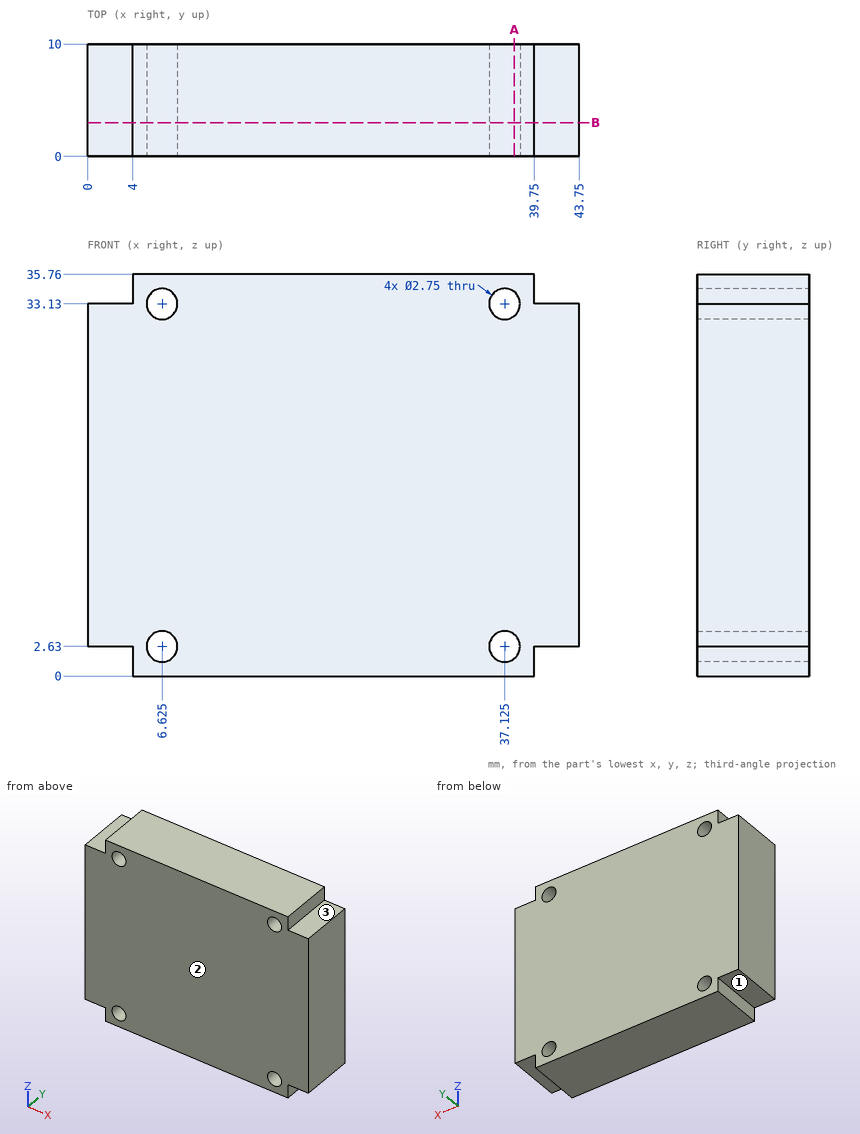
Print and shaded views of the part. All mm, measured from the part's lowest x, y and z. A direction names the side the tool comes from. Coordinates: 2 decimals unless noted, no trailing zeros. Order: outer loops, then holes, each group sorted by start corner. A loop starts at its lowest first (then second) coordinate and runs counter-clockwise, first axis right, second up. Notation, with made-up numbers: (84, -26.5) -> (95, -26.5) arc R22 cw to (95, -17.5) -> close; hole circle Ø11 at (3.25, 61.25). An arc over 180 degrees is marked (long way). Use one line per item in the form item = value. Start each with the question number.
1) Drill centre lines: L1, parallel to X at y = 1, z = 33; L2, parallel to X at y = 0.75, z = 3.5. Where is each one in solid material? Low to high. Write a range as [from, to].
2) Drop flat-ended pins along their axis: pin 1 (2 mm diameter, centred on y = 4.5, z = 0.5, fed in from +X); pin 2 (3 mm diameter, centred on y = 5, z = 0.5, fed in from -X); pin 3 (2 mm diameter, centred on x = 2, y = 5.5, fed in from -Z); pin 4 (2.5 mm diameter, centred on x = 6.625, z = 2.63, fed in from -Y). Give the stop position or say it passes through.
3) Band-saw the part on A-A on x = 38. Give the cut face in (y, z), then the cut area to 3 significant figures.
4) Tool access for the marked faces 1, 2 and 3: list every direction of +Z, -Z, +X, -X, +Y, -Y with a clear straight run to the whole face (end or side of a thin tool).
5) Band-saw the part on B-B on y = 3. Give the cut face in (x, z) (3 decimals).
Entries:
q1.L1 = [0, 5.26], [7.99, 35.76], [38.49, 43.75]
q1.L2 = [0, 5.56], [7.69, 36.06], [38.19, 43.75]
q2.pin_1 = 39.75
q2.pin_2 = 4
q2.pin_3 = 2.63
q2.pin_4 = through
q3.outline = (0, 0) -> (10, 0) -> (10, 1.57) -> (0, 1.57) -> close; (0, 3.69) -> (10, 3.69) -> (10, 32.07) -> (0, 32.07) -> close; (0, 34.19) -> (10, 34.19) -> (10, 35.76) -> (0, 35.76) -> close
q3.area = 315 mm2
q4.face_1 = -Z, -X, +Y, -Y
q4.face_2 = +Z, -Z, +X, -X, -Y
q4.face_3 = +Z, +X, +Y, -Y
q5.outline = (0, 2.63) -> (4, 2.63) -> (4, 0) -> (39.75, 0) -> (39.75, 2.63) -> (43.75, 2.63) -> (43.75, 33.13) -> (39.75, 33.13) -> (39.75, 35.76) -> (4, 35.76) -> (4, 33.13) -> (0, 33.13) -> close; hole circle Ø2.75 at (6.625, 2.63); hole circle Ø2.75 at (6.625, 33.13); hole circle Ø2.75 at (37.125, 2.63); hole circle Ø2.75 at (37.125, 33.13)
